Geometry: final body of the model. Coordinates: model frame, mm. A direction names the side the tool comes from. Give positions to 0.01 mm unless a question says otherwise; leave off trailing zeros. Write each loop counter-clockwise with the first axis right and the second up, starting at its lowest first coordinate (ties: lowest second). Pieces come first, ordered by that corner, then holes. Notation, with made-up numbers: M -26.5,41 L -17.5,41 A8 cw -17.5,47 Z; hole C -13.75,-18.75 d7. An arc over 180 degrees is marked long. Answer as a JSON object with one key per item and string values.
Autodesk Inventor part; units mm, degrees
ref_plane "YZ Plane" through (0, 0, 0) normal (1, 0, 0) x (0, 1, 0)
ref_plane "XZ Plane" through (0, 0, 0) normal (0, 1, 0) x (-1, 0, 0)
ref_plane "XY Plane" through (0, 0, 0) normal (0, 0, 1) x (1, 0, 0)
sketch "Sketch1" plane through (0, 0, 0) normal (1, 0, 0) x (0, 1, 0)
  line L0 (21, 21) -> (-21, 21)
  line L1 (-21, 21) -> (-21, -21)
  line L2 (-21, -21) -> (21, -21)
  line L3 (21, -21) -> (21, 21)
  point P0 (0, 0)
  point P1 (0, 21)
  point P2 (21, 0)
  dimension "d0" = 42
  dimension "d1" = 42
extrude "Extrusion1" add sketch "Sketch1" along normal blind 47
sketch "Sketch2" plane through (0, 0, 0) normal (-1, 0, 0) x (0, 0, 1)
  circle A0 centre (0, 0) radius 2.5
  dimension "d4" = 5
extrude "Extrusion2" add sketch "Sketch2" along normal blind 12
sketch "Sketch3" plane through (0, 0, 0) normal (-1, 0, 0) x (0, 0, 1)
  circle A0 centre (15.5, 15.5) radius 2
  line L0 (-13.7584, 0) -> (4.183, 0) construction
  line L1 (0, 11.541) -> (0, -2.5) construction
  circle A1 centre (0, 0) radius 2.5 construction
  circle A2 centre (15.5, -15.5) radius 2
  circle A3 centre (-15.5, 15.5) radius 2
  circle A4 centre (-15.5, -15.5) radius 2
  dimension "d7" = 15.5
  dimension "d8" = 15.5
  dimension "d9" = 4
extrude "Extrusion3" cut sketch "Sketch3" against normal blind 12
properties part number "NEMA 17 Completely Correct"
1) Pull-direction query (Y, two-part tool) for faces 3 (the flat face through (23, 21, 0)), 4 (the flat face through (12, 16, 15)), 5 (the flat face through (-12, 0, 0)), 6 (the flat face through (23, -21, 0)); classes: pulls with the +Y half, pulls with the -Y half, needs draft (parallel to the pull), parting line crosses it, or undercut.
Geometry check:
{"face 3": "pulls with the +Y half", "face 4": "undercut", "face 5": "needs draft", "face 6": "pulls with the -Y half"}
2) Cut plane A-A on y = 1.5. Return loops of the section in (x, z), and give its area (3 significant figures).
Geometry check:
{"outline": "M -12,-2 L 0,-2 L 0,-21 L 47,-21 L 47,21 L 0,21 L 0,2 L -12,2 Z", "area": "2,020 mm2"}
3) Contact query for flat-ended pins moving along their axis: P1, Ø1.2, axis at y = 15.5, z = 15, coming from the -X side; P2, Ø2, axis at y = -14.5, z = -16, coming from the -X side; P3, Ø5, axis at x = -1, y = 3.5, coming from the -Z side. Output: stop coordinate, or through.
Geometry check:
{"P1": "stops at x = 12", "P2": "stops at x = 0", "P3": "stops at z = -21"}
4) Set-up query: faces 1 (the flat face through (47, 0, 0)), 2 (the flat face through (12, -15, 15)). Return all of +Z, -Z, +X, -X, +Y, -Y with unobstructed straight access to the full face (end or side cutting, diameter ignored); none if empty.
Geometry check:
{"face 1": "+Z, -Z, +X, +Y, -Y", "face 2": "-X"}
5) Cut plane D-D on x = -7. Return loops of the section in (y, z), and give its area (3 significant figures).
Geometry check:
{"outline": "C 0,0 d5", "area": "19.6 mm2"}
6) Cut plane B-B on x = 2. Return loops of the section in (y, z).
Geometry check:
{"outline": "M -21,-21 L 21,-21 L 21,21 L -21,21 Z; hole C -15.5,-15.5 d4; hole C -15.5,15.5 d4; hole C 15.5,-15.5 d4; hole C 15.5,15.5 d4"}
7) Line query: line 1 (Y direction, x = 5.5, z = 15.5); line 2 (Z direction, x = 7, y = 15). Output: solid intervals per line, ascending. Write a range as from..to.
Geometry check:
{"line 1": "y = -21..-17.5, -13.5..13.5, 17.5..21", "line 2": "z = -21..-17.44, -13.56..13.56, 17.44..21"}
